from build123d import *

# Parameters (mm, degrees)
SKETCH1_W                 = 28.575
SKETCH1_H                 = 9.652
BOSS_EXTRUDE1_DEPTH       = 6.35
F_4_CLEARANCE_HOLE1_D     = 3.2639
F_4_CLEARANCE_HOLE2_D     = 3.2639
F_4_CLEARANCE_HOLE2_DEPTH = 23.8115
F_4_CLEARANCE_HOLE2_TIP   = 0.980574487


with BuildPart() as part:
    # Sketch1 → Boss-Extrude1 (new body)
    with BuildSketch(Plane.XY):
        Rectangle(SKETCH1_W, SKETCH1_H)
    extrude(amount=BOSS_EXTRUDE1_DEPTH)

    # #4 Clearance Hole1 (through all)
    with Locations(Plane.XY.offset(6.35)):
        with Locations((9.525, 0.0635)):
            Hole(F_4_CLEARANCE_HOLE1_D / 2)

    # #4 Clearance Hole2
    with Locations(Plane.ZY.offset(14.2875)):
        with Locations((3.175, 0)):
            Hole(F_4_CLEARANCE_HOLE2_D / 2, depth=F_4_CLEARANCE_HOLE2_DEPTH)
            with Locations((0, 0, -(F_4_CLEARANCE_HOLE2_DEPTH + F_4_CLEARANCE_HOLE2_TIP / 2))):  # 118° drill point
                Cone(0, F_4_CLEARANCE_HOLE2_D / 2, F_4_CLEARANCE_HOLE2_TIP, mode=Mode.SUBTRACT)


solid = part.part
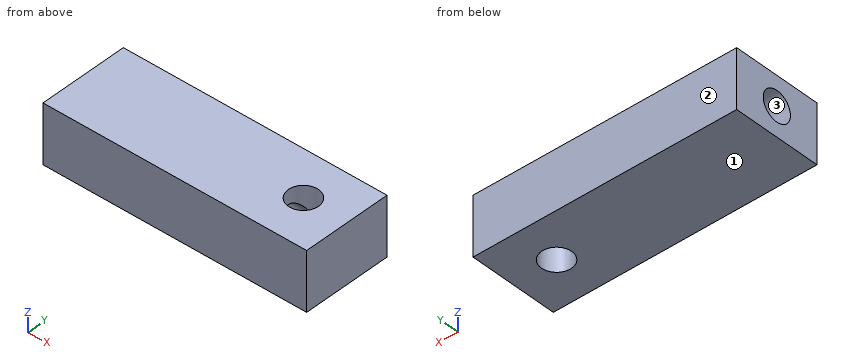
The model under review builds one solid part; all positions refer to its coordinate system, in mm. Face numbers are marked on the shaded views. Round coordinates to 2 decimals unless told otherwise and drop trailing zeros. Write each loop counter-clockwise with the first axis right and the second up, starting at its lowest first coordinate (ties: lowest second). Pieces come first, ordered by that corner, then holes. Notation, with made-up numbers: (77.25, 3.25) - (133.25, 3.25) arc R5 cw to (133.25, 7.25) - close; hole circle Ø6 at (75, 24). An arc over 180 degrees is marked (long way). One line per item, written item: value. Start each with the question number.
1. The part is to be moulded in two halves that separate along Z. For the marked faces 1, 2 and 3, say which applies: released by +Z, released by -Z, zero draft, split by the parting line, or undercut.
2. To check wall thickness, follow L1, parallel to Z at x = -4.5, y = 0; L2, parallel to Y at x = 5, z = 2; L3, parallel to Y at x = -3.25, z = 4. State the ranges of each line that lie inside material, in increasing order. Write a range as from..to.
3. Consider section D-D on z = 4.5. Write out the cut boundary in (x, y) (1 decimal), and give its area (3 significant figures).
4. Consider section A-A on y = 0.75. Write out the cut boundary in (x, z).
5. Clearance check with a flat-ended pin moving along its axis: P1, Ø1, axis at x = -9, y = -1.5, coming from the -Z side. State where the tip first meets the part, or that it passes through.
6. Consider section C-C on x = 9.25. Write out the cut boundary in (y, z) (3 decimals).
7. Consider section B-B on x = -4. Write out the cut boundary in (y, z) (3 decimals), and give its area (3 significant figures).
Checks:
1. face 1: released by -Z
1. face 2: zero draft
1. face 3: undercut
2. L1: z = 0..1.54, 4.81..6.35
2. L2: y = -4.83..-1.13, 1.13..4.83
2. L3: y = -4.83..-1.41, 1.41..4.83
3. outline: (-14.3, -4.8) - (14.3, -4.8) - (14.3, 4.8) - (-14.3, 4.8) - (-14.3, 1) - (8.2, 1) arc R1.6 cw (long way) to (8.2, -1) - (-14.3, -1) - close
3. area: 225 mm^2
4. outline: (-14.29, 0) - (8.04, 0) - (8.04, 1.73) - (-14.29, 1.73) - close; (-14.29, 4.62) - (8.04, 4.62) - (8.04, 6.35) - (-14.29, 6.35) - close; (11.01, 0) - (14.29, 0) - (14.29, 6.35) - (11.01, 6.35) - close
5. P1: stops at z = 0
6. outline: (-4.826, 0) - (-1.545, 0) - (-1.545, 2.65) arc R1.632 cw to (-1.545, 3.7) - (-1.545, 6.35) - (-4.826, 6.35) - close; (1.672, 0) - (4.826, 0) - (4.826, 6.35) - (1.672, 6.35) - close
7. outline: (-4.826, 0) - (4.826, 0) - (4.826, 6.35) - (-4.826, 6.35) - close; hole circle Ø3.264 at (0, 3.175)
7. area: 52.9 mm^2
